```python
from build123d import *

# Parameters (mm, degrees)
SKETCH1_W           = 100
SKETCH1_H           = 40
BOSS_EXTRUDE1_DEPTH = 5
CUT_EXTRUDE1_DEPTH  = 5
CUT_EXTRUDE2_DEPTH  = 5
CUT_EXTRUDE3_DEPTH  = 5
CUT_EXTRUDE4_DEPTH  = 5
SKETCH3_W           = 70
SKETCH3_H           = 25
BOSS_EXTRUDE2_DEPTH = 100
FILLET1_R           = 5
FILLET2_R           = 2.5
CUT_EXTRUDE8_DEPTH  = 28.5
FILLET3_R           = 2.5
CUT_EXTRUDE9_DEPTH  = 28.5
CUT_EXTRUDE10_REACH = 107
SKETCH10_R          = 3.25


with BuildPart() as part:
    # Sketch1 → Boss-Extrude1 (new body)
    with BuildSketch(Plane.XY):
        Rectangle(SKETCH1_W, SKETCH1_H)
    extrude(amount=BOSS_EXTRUDE1_DEPTH)

    # Sketch2 → Cut-Extrude1 (cut)
    with BuildSketch(Plane.XY.offset(5)):
        with BuildLine():
            Line((-40.25, 17), (-40.25, -13))
            ThreePointArc((-40.25, -13), (-42.5, -15.25), (-44.75, -13))
            Line((-44.75, -13), (-44.75, 17))
            ThreePointArc((-44.75, 17), (-42.5, 19.25), (-40.25, 17))
        make_face()
    extrude(amount=-CUT_EXTRUDE1_DEPTH, mode=Mode.SUBTRACT)

    # Sketch2_3 → Cut-Extrude2 (cut)
    with BuildSketch(Plane.XY.offset(5)):
        with BuildLine():
            Line((-35, -10.75), (-5, -10.75))
            ThreePointArc((-5, -10.75), (-2.75, -13), (-5, -15.25))
            Line((-5, -15.25), (-35, -15.25))
            ThreePointArc((-35, -15.25), (-37.25, -13), (-35, -10.75))
        make_face()
    extrude(amount=-CUT_EXTRUDE2_DEPTH, mode=Mode.SUBTRACT)

    # Sketch2_4 → Cut-Extrude3 (cut)
    with BuildSketch(Plane.XY.offset(5)):
        with BuildLine():
            Line((5, -10.75), (35, -10.75))
            ThreePointArc((35, -10.75), (37.25, -13), (35, -15.25))
            Line((35, -15.25), (5, -15.25))
            ThreePointArc((5, -15.25), (2.75, -13), (5, -10.75))
        make_face()
    extrude(amount=-CUT_EXTRUDE3_DEPTH, mode=Mode.SUBTRACT)

    # Sketch2_5 → Cut-Extrude4 (cut)
    with BuildSketch(Plane.XY.offset(5)):
        with BuildLine():
            Line((44.75, 17), (44.75, -13))
            ThreePointArc((44.75, -13), (42.5, -15.25), (40.25, -13))
            Line((40.25, -13), (40.25, 17))
            ThreePointArc((40.25, 17), (42.5, 19.25), (44.75, 17))
        make_face()
    extrude(amount=-CUT_EXTRUDE4_DEPTH, mode=Mode.SUBTRACT)

    # Sketch3 → Boss-Extrude2 (add)
    with BuildSketch(Plane.XY.offset(5)):
        with Locations((0, 5)):
            Rectangle(SKETCH3_W, SKETCH3_H)
    extrude(amount=BOSS_EXTRUDE2_DEPTH)

    # Fillet1
    fillet1_edges = [part.edges().sort_by_distance(p)[0] for p in [
        (-50, 20, 2.5),
        (50, 20, 2.5),
        (50, -20, 2.5),
        (-50, -20, 2.5),
    ]]
    fillet(fillet1_edges, radius=FILLET1_R)

    # Fillet2
    fillet2_edges = [part.edges().sort_by_distance(p)[0] for p in [
        (-35, 17.5, 55),
        (-35, -7.5, 55),
        (35, -7.5, 55),
        (35, 17.5, 55),
    ]]
    fillet(fillet2_edges, radius=FILLET2_R)

    # Sketch8 → Cut-Extrude8 (cut, through all)
    with BuildSketch(Plane.XZ.offset(7.5)):
        Polygon((-28.75, 9), (28.75, 9), (28.75, 64.875885604), (0, 89), (-28.75, 64.875885604), align=None)
    extrude(amount=-CUT_EXTRUDE8_DEPTH, mode=Mode.SUBTRACT)

    # Fillet3
    fillet3_edges = [part.edges().sort_by_distance(p)[0] for p in [
        (28.75, 5, 9),
        (-28.75, 5, 9),
        (-28.75, 5, 64.875885604),
        (28.75, 5, 64.875885604),
    ]]
    fillet(fillet3_edges, radius=FILLET3_R)

    # Sketch9 → Cut-Extrude9 (cut, through all)
    with BuildSketch(Plane.XZ.offset(7.5)):
        Polygon((-30, 94.061848056), (-30, 84.061848056), (-15, 84.061848056), (-15, 94.061848056), (-22.5, 103), align=None)
        Polygon((15, 94.061848056), (22.5, 103), (30, 94.061848056), (30, 84.061848056), (15, 84.061848056), align=None)
    extrude(amount=-CUT_EXTRUDE9_DEPTH, mode=Mode.SUBTRACT)

    # Sketch10 → Cut-Extrude10 (cut, up to next)
    with BuildSketch(Plane.XY.offset(105), mode=Mode.PRIVATE) as cut_extrude10_sk1:
        with Locations((-22.252451, 5)):
            Circle(SKETCH10_R)
    cut_extrude10_tool1 = extrude(cut_extrude10_sk1.sketch, amount=-CUT_EXTRUDE10_REACH, mode=Mode.PRIVATE) & part.part
    add(cut_extrude10_tool1.solids().sort_by_distance((-22.252451, 5, 105))[0], mode=Mode.SUBTRACT)
    # Sketch10 → Cut-Extrude10 (cut, up to next)
    with BuildSketch(Plane.XY.offset(105), mode=Mode.PRIVATE) as cut_extrude10_sk2:
        with Locations((22.252451, 5)):
            Circle(SKETCH10_R)
    cut_extrude10_tool2 = extrude(cut_extrude10_sk2.sketch, amount=-CUT_EXTRUDE10_REACH, mode=Mode.PRIVATE) & part.part
    add(cut_extrude10_tool2.solids().sort_by_distance((22.252451, 5, 105))[0], mode=Mode.SUBTRACT)


solid = part.part
```
Design review of the part built by this model. Coordinates are the model's own, in mm. A direction names the side the tool comes from. Coordinates: 2 decimals unless noted, no trailing zeros. Write each loop counter-clockwise with the first axis right and the second up, starting at its lowest first coordinate (ties: lowest second). Pieces come first, ordered by that corner, then holes.
1) Add section B-B (x = -42.5). Write out the cut boundary in (y, z).
2) Add section A-A (y = -9.5). Write out the cut boundary in (x, z), plus the area to 3 significant figures.
3) Add section D-D (x = -21). Write out the cut boundary in (y, z).
4) Add section C-C (z = 45). Write out the cut boundary in (x, y), plus the area to 3 significant figures.
5) Machinability: for faces 4 (the flat face through (28.75, 5, 37)), 5 (the cylindrical face through (-2.75, -12.95, 2.54)), 6 (the flat face through (-15, 17.5, 77)), which of the approach directions +Z, -Z, +X, -X, +Y, -Y give a long, thin tool a straight path to every point of the face, cutting with its end or side? Answer none if there is none.
6) Insertion check: pin 1 (12.5 mm diameter, centred on y = 4.5, z = 25, fed in from +X); pin 2 (16 mm diameter, centred on y = 9, z = 75, fed in from -X); pin 3 (10 mm diameter, centred on x = 29.5, z = 16.5, fed in from -Y). Each pin has a flat end and moves straight along its axis. Give the tip position at first contact, or say it passes through.
7) Mouldability with a two-part tool opening along Z and no side actions: class faces 1 (the flat face through (-30, 5, 89)), 2 (the flat face through (23, 5, 84.062)), 3 (the cylindrical face through (-37.25, -13.05, 2.54)) as +Z half, -Z half, draft (parallel to the pull), parting line (faces both ways), or undercut.
8) To check wall thickness, follow L1, parallel to X at y = 5, z = 103; L2, parallel to Z at x = -46, y = -5.5; L3, parallel to X at y = 10.5, z = 94.5. State the ranges of each line that lie inside material, in increasing order.
Check result:
1. outline: (-20, 0) - (-15.25, 0) - (-15.25, 5) - (-20, 5) - close; (19.25, 0) - (20, 0) - (20, 5) - (19.25, 5) - close
2. outline: (-50, 0) - (-44.75, 0) - (-44.75, 5) - (-50, 5) - close; (-40.25, 0) - (40.25, 0) - (40.25, 5) - (-40.25, 5) - close; (44.75, 0) - (50, 0) - (50, 5) - (44.75, 5) - close
2. area: 455 mm2
3. outline: (-20, 0) - (-15.25, 0) - (-15.25, 5) - (-20, 5) - close; (-10.75, 0) - (20, 0) - (20, 5) - (17.5, 5) - (17.5, 9) - (-7.5, 9) - (-7.5, 5) - (-10.75, 5) - close; (-7.5, 71.38) - (17.5, 71.38) - (17.5, 84.06) - (-7.5, 84.06) - close; (-7.5, 101.21) - (2, 101.21) - (2, 105) - (-7.5, 105) - close; (8, 101.21) - (17.5, 101.21) - (17.5, 105) - (8, 105) - close
4. outline: (-35, -5) arc R2.5 ccw to (-32.5, -7.5) - (-28.75, -7.5) - (-28.75, 17.5) - (-32.5, 17.5) arc R2.5 ccw to (-35, 15) - close; (28.75, -7.5) - (32.5, -7.5) arc R2.5 ccw to (35, -5) - (35, 15) arc R2.5 ccw to (32.5, 17.5) - (28.75, 17.5) - close
4. area: 307 mm2
5. face 4: +Y, -Y
5. face 5: +Z, -Z
5. face 6: +Z, +X, -X, +Y
6. pin 1: stops at x = 35
6. pin 2: stops at x = -35
6. pin 3: stops at y = -7.5
7. face 1: undercut
7. face 2: undercut
7. face 3: draft
8. L1: x = -35 to -25.5, -19 to 19, 25.5 to 35
8. L2: z = 0 to 5
8. L3: x = -35 to -29.63, -15.37 to 15.37, 29.63 to 35
